from build123d import *

# Parameters (mm, degrees)
SKETCH2_W           = 15
SKETCH2_H           = 15
SKETCH2_W_2         = 30
SKETCH2_R           = 4
BOSS_EXTRUDE1_DEPTH = 10
SKETCH2_3_W         = 15
SKETCH2_3_H         = 15
SKETCH2_3_W_2       = 30
SKETCH2_3_R         = 4
BOSS_EXTRUDE2_DEPTH = 10
SKETCH4_R           = 1.6
CUT_EXTRUDE1_DEPTH  = 16
CUT_EXTRUDE2_START  = -6.25
SKETCH4_3_R         = 1.6
CUT_EXTRUDE2_DEPTH  = 2.5


with BuildPart() as part:
    # Sketch2 → Boss-Extrude1 (new body)
    with BuildSketch(Plane(origin=(0, 0, 0), x_dir=(1, 0, 0), z_dir=(0, 1, 0))):
        with Locations((-22.5, 0)):
            Rectangle(SKETCH2_W, SKETCH2_H)
        Rectangle(SKETCH2_W_2, SKETCH2_H)
        with Locations((7.5, 0)):
            Circle(SKETCH2_R, mode=Mode.SUBTRACT)
        with Locations((-7.5, 0)):
            Circle(SKETCH2_R, mode=Mode.SUBTRACT)
        with Locations((22.5, 0)):
            Rectangle(SKETCH2_W, SKETCH2_H)
    extrude(amount=BOSS_EXTRUDE1_DEPTH)

    # Sketch2_3 → Boss-Extrude2 (add)
    with BuildSketch(Plane(origin=(0, 0, 0), x_dir=(1, 0, 0), z_dir=(0, 1, 0))):
        with Locations((-22.5, 0)):
            Rectangle(SKETCH2_3_W, SKETCH2_3_H)
        Rectangle(SKETCH2_3_W_2, SKETCH2_3_H)
        with Locations((7.5, 0)):
            Circle(SKETCH2_3_R, mode=Mode.SUBTRACT)
        with Locations((-7.5, 0)):
            Circle(SKETCH2_3_R, mode=Mode.SUBTRACT)
        with Locations((-7.5, 0)):
            Circle(SKETCH2_3_R)
        with Locations((7.5, 0)):
            Circle(SKETCH2_3_R)
        with Locations((22.5, 0)):
            Rectangle(SKETCH2_3_W, SKETCH2_3_H)
    extrude(amount=-BOSS_EXTRUDE2_DEPTH)

    # Sketch4 → Cut-Extrude1 (cut, through all)
    with BuildSketch(Plane.XY.offset(7.5)):
        with Locations((-22.5, -5)):
            Circle(SKETCH4_R)
        with Locations((-22.5, 5)):
            Circle(SKETCH4_R)
        with Locations((22.5, 5)):
            Circle(SKETCH4_R)
        with Locations((22.5, -5)):
            Circle(SKETCH4_R)
    extrude(amount=-CUT_EXTRUDE1_DEPTH, mode=Mode.SUBTRACT)

    # Sketch4_3 → Cut-Extrude2 (cut)
    with BuildSketch(Plane.XY.offset(7.5).offset(CUT_EXTRUDE2_START)):
        Polygon((-22.5, 8.435234102), (-25.475, 6.717617051), (-25.475, 3.282382949), (-22.5, 1.564765898), (-19.525, 3.282382949), (-19.525, 6.717617051), align=None)
        with Locations((-22.5, 5)):
            Circle(SKETCH4_3_R, mode=Mode.SUBTRACT)
        Polygon((22.5, 8.435234102), (19.525, 6.717617051), (19.525, 3.282382949), (22.5, 1.564765898), (25.475, 3.282382949), (25.475, 6.717617051), align=None)
        with Locations((22.5, 5)):
            Circle(SKETCH4_3_R, mode=Mode.SUBTRACT)
        Polygon((-22.5, -8.435234102), (-19.525, -6.717617051), (-19.525, -3.282382949), (-22.5, -1.564765898), (-25.475, -3.282382949), (-25.475, -6.717617051), align=None)
        with Locations((-22.5, -5)):
            Circle(SKETCH4_3_R, mode=Mode.SUBTRACT)
        Polygon((22.5, -8.435234102), (25.475, -6.717617051), (25.475, -3.282382949), (22.5, -1.564765898), (19.525, -3.282382949), (19.525, -6.717617051), align=None)
        with Locations((22.5, -5)):
            Circle(SKETCH4_3_R, mode=Mode.SUBTRACT)
    extrude(amount=-CUT_EXTRUDE2_DEPTH, mode=Mode.SUBTRACT)


solid = part.part
CAD build for the part. Positions are in the model's coordinates, mm. A direction names the side the tool comes from. Give positions to 0.01 mm unless a question says otherwise; leave off trailing zeros. Loops run counter-clockwise (first coordinate to the right, second up) from the corner with the lowest first, then second, coordinate; pieces in that order, holes last. Notation, with made-up numbers: M -2.75,-2.75 L 47.25,-2.75 A9 ccw 47.25,1.25 Z; hole C 25.25,71 d6. An arc over 180 degrees is marked long. Answer in a Markdown table with one row per item. Add a question column.
Item 1: Mould opens along Z. For faces 3 (the face through (-24.008, -7.564, 0.018)), 4 (the face through (0, 0, 7.5)), 5 (the face through (-21.76, 3.58, -4.33)) say: +Z half, -Z half, draft (parallel to the pull), parting line (faces both ways), or undercut.
Item 2: Band-saw the part on C-C on y = -5. Give the cut face in (x, z) (3 decimals), then the cut area to 3 significant figures.
Item 3: Drop a flat-ended pin along its axis: P1, Ø3, axis at x = -22.5, y = 5, coming from the +Z side. Give the stop position or say it passes through.
Item 4: Tool access for faces 1 (the face through (23.24, 3.58, 4.42)), 2 (the face through (24, 4, 1.25)): list every direction of +Z, -Z, +X, -X, +Y, -Y with a clear straight run to the whole face (end or side of a thin tool).
Item 5: Band-saw the part on B-B on z = 5.75. Give the cut face in (x, y), then the cut area to 3 significant figures.
Item 6: Band-saw the part on D-D on x = -7.5. Give the cut face in (y, z).
Item 7: Probe probe 1 along Y at (x, z) = (-22.5, -5.25); probe 2 along X at (y, z) = (6.5, 0) (3 decimals); probe 3 along Z at (x, y) = (-22.5, -7.75). List the from-to ranges inside material, lowest first.
Item 8: Band-saw the part on A-A on y = 5. Give the number of separate pieces and of enclosed holes in the cut face, then the cut area to 3 significant figures.
Reply:
| question | item | result |
|---|---|---|
| 1 | face 3 | undercut |
| 1 | face 4 | +Z half |
| 1 | face 5 | draft |
| 2 | outline | M -30,-7.5 L -24.1,-7.5 L -24.1,-1.25 L -25.475,-1.25 L -25.475,1.25 L -24.1,1.25 L -24.1,7.5 L -30,7.5 Z; M -20.9,-7.5 L 20.9,-7.5 L 20.9,-1.25 L 19.525,-1.25 L 19.525,1.25 L 20.9,1.25 L 20.9,7.5 L -20.9,7.5 L -20.9,1.25 L -19.525,1.25 L -19.525,-1.25 L -20.9,-1.25 Z; M 24.1,-7.5 L 30,-7.5 L 30,7.5 L 24.1,7.5 L 24.1,1.25 L 25.475,1.25 L 25.475,-1.25 L 24.1,-1.25 Z |
| 2 | area | 790 mm^2 |
| 3 | P1 | passes through |
| 4 | face 1 | +Z, -Z |
| 4 | face 2 | none |
| 5 | outline | M -30,-10 L 30,-10 L 30,10 L -30,10 Z; hole C -22.5,-5 d3.2; hole C -22.5,5 d3.2; hole C 22.5,-5 d3.2; hole C 22.5,5 d3.2 |
| 5 | area | 1,170 mm^2 |
| 6 | outline | M -10,-7.5 L 10,-7.5 L 10,-4 L 0,-4 L 0,4 L 10,4 L 10,7.5 L -10,7.5 Z |
| 7 | probe 1 | y = -10 to -6.6, -3.4 to 3.4, 6.6 to 10 |
| 7 | probe 2 | x = -30 to -25.475, -19.525 to -11.5, -3.5 to 3.5, 11.5 to 19.525, 25.475 to 30 |
| 7 | probe 3 | z = -7.5 to -1.25, 1.25 to 7.5 |
| 8 | separate pieces | 3 |
| 8 | enclosed holes | 2 |
| 8 | area | 690 mm^2 |
